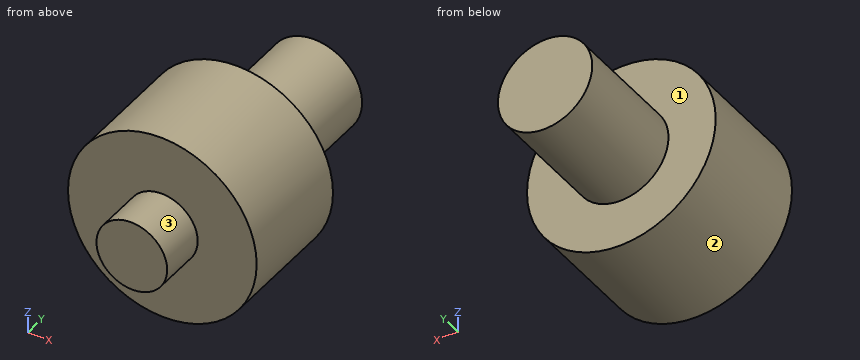
from build123d import *

# Parameters (mm, degrees)
F0_R     = 8
F1_DEPTH = 24
F2_R     = 12.156752
F2_R_2   = 3
F3_DEPTH = 4
F4_R     = 10.910095
F4_R_2   = 4
F5_DEPTH = 10


with BuildPart() as f1:
    # F0 (on Front) → F1 (new body)
    with BuildSketch(Plane.XZ):
        Circle(F0_R)
    extrude(amount=-F1_DEPTH)

    # F2 (on face) → F3 (cut)
    with BuildSketch(Plane.XZ):
        Circle(F2_R)
        Circle(F2_R_2, mode=Mode.SUBTRACT)
    extrude(amount=-F3_DEPTH, mode=Mode.SUBTRACT)

    # F4 (on face) → F5 (cut)
    with BuildSketch(Plane(origin=(0, 24, 0), x_dir=(-1, 0, 0), z_dir=(0, 1, 0))):
        Circle(F4_R)
        Circle(F4_R_2, mode=Mode.SUBTRACT)
    extrude(amount=-F5_DEPTH, mode=Mode.SUBTRACT)


solid = f1.part
Geometry: final body of the model. Coordinates: model frame, mm. Face numbers are marked on the shaded views. A direction names the side the tool comes from. Round coordinates to 2 decimals unless told otherwise and drop trailing zeros. Order: outer loops, then holes, each group sorted by start corner. A loop starts at its lowest first (then second) coordinate and runs counter-clockwise, first axis right, second up.
Q1. Access query for the marked faces 1, 2 and 3. Directions: +Z, -Z, +X, -X, +Y, -Y. A direction counts if a zero-diameter tool reaches every point of the face in a straight line with its end or side. Return the directions, or none.
Result sheet:
face 1: +Y
face 2: +Y, -Y
face 3: -Y
Q2. Pin query (flat end, axial travel): pin 1 (2 mm diameter, centred on x = -5.5, y = 15.5, fed in from -Z); pin 2 (2 mm diameter, centred on x = -5, z = 0.5, fed in from -Y); pin 3 (8 mm diameter, centred on x = -3, y = 20, fed in from +Z); pin 4 (6 mm diameter, centred on y = 7.5, z = 3.5, fed in from -X). Return the tip coordinate at first contact, or that it passes through.
Result sheet:
pin 1: passes through
pin 2: stops at y = 4
pin 3: stops at z = 4
pin 4: stops at x = -7.98
Q3. Section A-A, the plane x = 0. Output: boundary loops of the cut face in (y, z), and give its area (3 significant figures).
Result sheet:
outline: (0, -3) - (4, -3) - (4, -8) - (14, -8) - (14, -4) - (24, -4) - (24, 4) - (14, 4) - (14, 8) - (4, 8) - (4, 3) - (0, 3) - close
area: 264 mm2
Q4. Section D-D, the plane x = -3.5. Output: boundary loops of the cut face in (y, z).
Result sheet:
outline: (4, -7.19) - (14, -7.19) - (14, -1.94) - (24, -1.94) - (24, 1.94) - (14, 1.94) - (14, 7.19) - (4, 7.19) - close
Q5. Section C-C, the plane y = 9. Output: boundary loops of the cut face in (x, z), and give its area (3 significant figures).
Result sheet:
outline: circle Ø16 at (0, 0)
area: 201 mm2
Q6. Material intervals for probe 1 along Y at (x, z) = (-2.5, 3); probe 2 along Y at (x, z) = (3.5, 4.25); probe 3 along Z at (x, y) = (6, 6.25), sorted ascending.
Result sheet:
probe 1: y = 4 to 24
probe 2: y = 4 to 14
probe 3: z = -5.29 to 5.29
Q7. Section B-B, the plane z = 0. Output: boundary loops of the cut face in (x, y), and give its area (3 significant figures).
Result sheet:
outline: (-8, 4) - (-3, 4) - (-3, 0) - (3, 0) - (3, 4) - (8, 4) - (8, 14) - (4, 14) - (4, 24) - (-4, 24) - (-4, 14) - (-8, 14) - close
area: 264 mm2
